from build123d import *

# Parameters (mm, degrees)
F1_DEPTH  = 19.05
F3_DEPTH  = 38.1
F5_DEPTH  = 38.1
F7_DEPTH  = 19.05
F9_DEPTH  = 57.15
F10_DEPTH = 38.1
F11_W     = 19.05
F11_H     = 38.1
F12_DEPTH = 25.4
F13_W     = 19.05
F13_H     = 19.05
F13_H_2   = 6.35
F14_DEPTH = 25.4
F15_DEPTH = 38.1


# Not quite as in the source:
# - a feature names something its author has since deleted; it is built from what else it names


with BuildPart() as f1:
    # F0 (on Right) → F1 (new body)
    with BuildSketch(Plane.YZ):
        Polygon((-19.05, 0), (0, 0), (0, 50.8), (-477.8375, 50.8), (-477.8375, 12.7), (-11.7176515813, 12.7), align=None)
    extrude(amount=F1_DEPTH)

    # F2 (on face) → F3 (join)
    with BuildSketch(Plane.YZ.offset(19.05)):
        Polygon((0, 12.7), (-11.7176515813, 12.7), (-19.05, 0), (0, 0), align=None)
    extrude(amount=F3_DEPTH)

    # F4 (on face) → F5 (join)
    with BuildSketch(Plane(origin=(0, 0, 0), x_dir=(0, -1, 0), z_dir=(-1, 0, 0))):
        Polygon((19.05, 0), (11.7176515813, 12.7), (0, 12.7), (0, 0), align=None)
    extrude(amount=F5_DEPTH)

    # F6 (on face) → F7 (join)
    with BuildSketch(Plane(origin=(0, 0, 0), x_dir=(-1, 0, 0), z_dir=(0, 1, 0))):
        Polygon((0, 50.8), (-19.05, 50.8), (-19.05, 12.7), (-19.05, 0), (0, 0), (0, 12.7), align=None)
    extrude(amount=F7_DEPTH)

    # F8 (on face) → F9 (join)
    with BuildSketch(Plane.YZ.offset(19.05)):
        Polygon((-462.9448484187, 12.7), (-473.075, 12.7), (-480.4073484187, 0), (-462.9448484187, 0), align=None)
    extrude(amount=-F9_DEPTH)

    # F8 (on face) → F10 (join)
    with BuildSketch(Plane.YZ.offset(19.05)):
        Polygon((-462.9448484187, 12.7), (-473.075, 12.7), (-480.4073484187, 0), (-462.9448484187, 0), align=None)
    extrude(amount=F10_DEPTH)

    # F11 (on face) → F12 (join)
    with BuildSketch(Plane.XZ.offset(477.8375)):
        with Locations((9.525, 31.75)):
            Rectangle(F11_W, F11_H)
    extrude(amount=F12_DEPTH)

    # F13 (on face) → F14 (join)
    with BuildSketch(Plane(origin=(0, 0, 12.7), x_dir=(1, 0, 0), z_dir=(0, 0, -1))):
        with Locations((9.525, 512.7625)):
            Rectangle(F13_W, F13_H)
        with Locations((9.525, 500.0625)):
            Rectangle(F13_W, F13_H_2)
    extrude(amount=F14_DEPTH)

    # F15 (add, through all): a face of the model
    f15_faces = [f1.faces().sort_by_distance(p)[0] for p in [
        (9.525, -512.7625, 12.7),
    ]]
    extrude(f15_faces, amount=F15_DEPTH)


solid = f1.part
Geometry check sheet. Reference: the model listing, model coordinates, mm. A direction names the side the tool comes from. Round coordinates to 2 decimals unless told otherwise and drop trailing zeros. Order: outer loops, then holes, each group sorted by start corner. A loop starts at its lowest first (then second) coordinate and runs counter-clockwise, first axis right, second up. Notation, with made-up numbers: M 58.5,-37.75 L 69.5,-37.75 A20 cw 69.5,-21.75 Z; hole C -25.5,36.25 d6. An arc over 180 degrees is marked long. Write each question's results on one line, items separated by ' | '. Start each with the question number.
1. Draft check along Y on faces 6 (the face through (9, -240, 12.7)), 7 (the face through (-38.1, -7, 6)), 8 (the face through (10, 19.05, 26)). Enter one of: pulls with the +Y half, pulls with the -Y half, needs draft (parallel to the pull), parting line crosses it, or undercut.
2. Cross-section at B-B on z = -6. Record the boundary of the cut face in (x, y).
3. Cross-section at C-C on y = -90.5. Record the boundary of the cut face in (x, z).
4. Cross-section at A-A on x = -28. Record the boundary of the cut face in (y, z) (3 decimals), plus the area to 3 significant figures.
5. Set-up check for faces 1 (the face through (-19, 0, 6)), 2 (the face through (10, -9, 0)), 3 (the face through (38, -6, 12.7)), 4 (the face through (-19, -468, 12.7)), 5 (the face through (9, -485, 12.7)): record each of +Z, -Z, +X, -X, +Y, -Y from which the full face is reachable in a straight line by a thin tool's end or side.
6. Go/stop test with flat-tipped pins: P1, Ø12, axis at x = -6.5, z = 14.5, coming from the -Y side; P2, Ø5, axis at x = 40.5, y = -469, coming from the +Z side; P3, Ø5.5, axis at x = 8.5, z = -4.5, coming from the +Y side. Record where each tip stops, or that it passes through.
7. Material ranges on L1, parallel to Y at x = 17, z = 3; L2, parallel to X at y = -456, z = 47.5; L3, parallel to Y at x = 9, z = -4, recorded low to high. Write a range as from..to.
Resolved:
1) face 6: undercut | face 7: needs draft | face 8: pulls with the +Y half
2) outline: M 0,-522.29 L 19.05,-522.29 L 19.05,-496.89 L 0,-496.89 Z
3) outline: M 0,12.7 L 19.05,12.7 L 19.05,50.8 L 0,50.8 Z
4) outline: M -480.407,0 L -462.945,0 L -462.945,12.7 L -473.075,12.7 Z; M -19.05,0 L 0,0 L 0,12.7 L -11.718,12.7 Z | area: 371 mm2
5) face 1: +Z, -Z, -X, +Y | face 2: -Z, +X, -X, +Y | face 3: +Z, +X, +Y, -Y | face 4: +Z, -X, +Y, -Y | face 5: +X, -X
6) P1: y = -475.5 | P2: z = 12.7 | P3: y = -496.89
7) L1: -522.29..-496.89, -478.68..-462.94, -17.32..19.05 | L2: 0..19.05 | L3: -522.29..-496.89
